Source: three-view drawing plus pictorial views. Frame: mm from the lowest corner of the part. A direction names the side the tool comes from. Give positions to 0.01 mm unless a question says otherwise; leave off trailing zeros. Loops run counter-clockwise (first coordinate to the right, second up) from the corner with the lowest first, then second, coordinate; pieces in that order, holes last. Notation, with made-up numbers: (-23, -8) - (-7, -8) arc R17 cw to (-7, 9) - close; hole circle Ø4 at (-27.5, 61.5). An arc over 180 degrees is marked (long way). Answer as a JSON object with one key per item and string values.
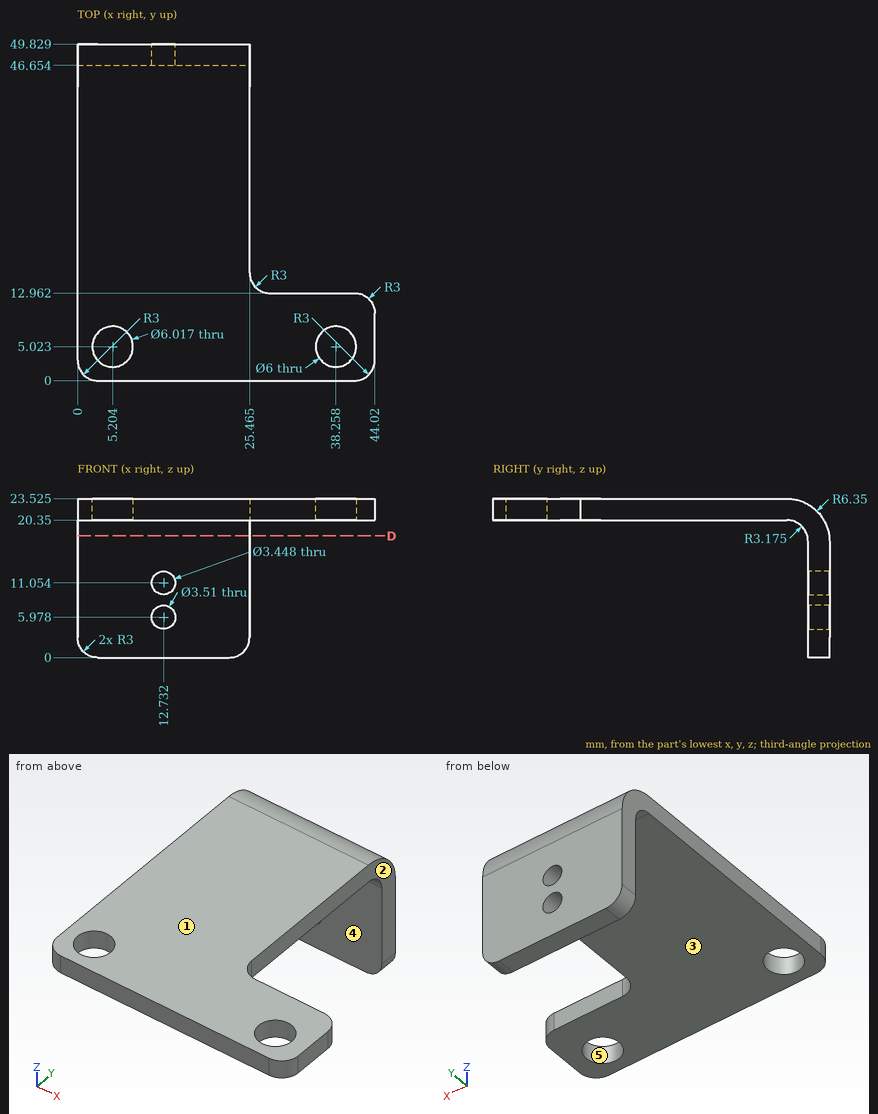
Item 1: Mould query, pull axis Y, two halves, no side actions, for the marked faces 3, 4 and 5. Classes: released by +Y, released by -Y, zero draft, split by the parting line, or undercut.
Geometry check:
{"face 3": "zero draft", "face 4": "released by -Y", "face 5": "undercut"}
Item 2: Material intervals for line 1 (Y direction, x = 38, z = 21.75); line 2 (Y direction, x = 10, z = 9); line 3 (X direction, y = 24, z = 22.75) (1 decimal), sorted ascending. Write a range as [from, to].
Geometry check:
{"line 1": "y = [0, 2.03], [8.01, 12.96]", "line 2": "y = [46.65, 49.83]", "line 3": "x = [0, 25.5]"}
Item 3: Contact query for flat-ended pins moving along their axis: P1, Ø9.5, axis at x = 5.2, y = 5.02, coming from the -Z side; P2, Ø1.6, axis at x = 32, z = 22.5, coming from the +Y side; P3, Ø8.5, axis at x = 16.5, z = 5, coming from the -Y side. Output: stop coordinate, or through.
Geometry check:
{"P1": "stops at z = 20.35", "P2": "stops at y = 12.96", "P3": "stops at y = 46.65"}
Item 4: Cut plane D-D (z = 18). Return loops of the section in (x, y) (1 decimal).
Geometry check:
{"outline": "(0, 46.5) - (25.5, 46.5) - (25.5, 49.8) - (0, 49.8) - close"}
Item 5: Access query for the marked faces 1 and 2. Directions: +Z, -Z, +X, -X, +Y, -Y. A direction counts if a zero-diameter tool reaches every point of the face in a straight line with its end or side. Return the directions, or none.
Geometry check:
{"face 1": "+Z, +X, -X, +Y, -Y", "face 2": "+Z, -Z, +X, +Y"}
